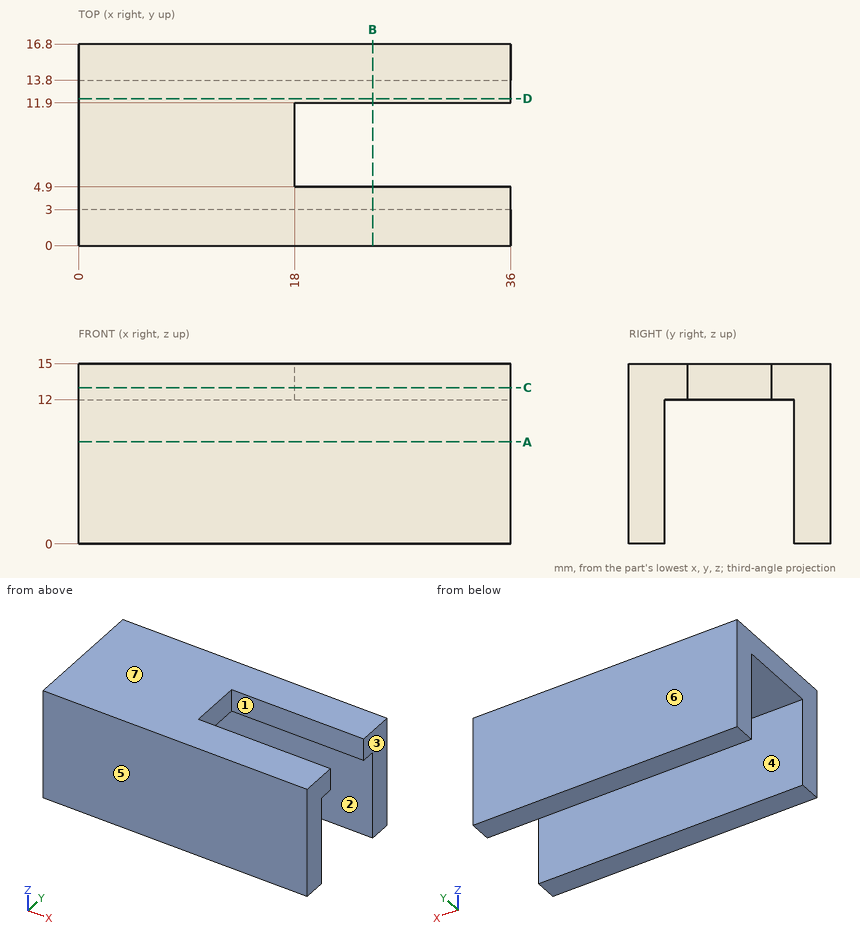
The figure shows three views and two pictorial views of one solid part (mm, origin at its lowest corner). Answer the questions. A direction names the side the tool comes from. Round coordinates to 2 decimals unless told otherwise and drop trailing zeros. Order: outer loops, then holes, each group sorted by start corner. A loop starts at its lowest first (then second) coordinate and runs counter-clockwise, first axis right, second up. Notation, with made-up numbers: (84.5, 27.25) - (93.5, 27.25) arc R11 cw to (93.5, 41.25) - close; hole circle Ø2 at (86.5, 67). An arc over 180 degrees is marked (long way). Write item = value, one per line. Start each with the question number.
1) Straight lines are drawn through the part: L1, parallel to Y at x = 33, z = 7.25; L2, parallel to Z at x = 9, y = 7.25; L3, parallel to X at y = 11.75, z = 13. For each, find the intervals that lie inside material, in ascending order.
2) Section C-C, the plane z = 13 is taken. Write down the section's boundary in (x, y).
3) Section D-D, the plane y = 12.25 is taken. Write down the section's boundary in (x, z).
4) Section B-B, the plane x = 24.5 is taken. Write down the section's boundary in (y, z).
5) Given pin 1 (1.5 mm diameter, centred on y = 7, z = 13, fed in from +X); pin 2 (1 mm diameter, centred on y = 12, z = 6, fed in from +X), each flat-ended and moving along its own axis, determine where each tip first touches the part or whether it passes through.
6) For a pull along Y with two mould halves and no side action, classify the marked faces 4, 5, 6 and 7 as released by +Y, released by -Y, zero draft, split by the parting line, or undercut.
7) For the marked faces 1, 2 and 3, determine the directions among +Z, -Z, +X, -X, +Y, -Y from which every point of the face is accessible in a straight line to the end or side of a thin tool.
8) Section A-A, the plane z = 8.5 is taken. Write down the section's boundary in (x, y), plus the area to 3 significant figures.
Results list:
q1.L1 = 0 to 3, 13.8 to 16.8
q1.L2 = 12 to 15
q1.L3 = 0 to 18
q2.outline = (0, 0) - (36, 0) - (36, 4.9) - (18, 4.9) - (18, 11.9) - (36, 11.9) - (36, 16.8) - (0, 16.8) - close
q3.outline = (0, 12) - (36, 12) - (36, 15) - (0, 15) - close
q4.outline = (0, 0) - (3, 0) - (3, 12) - (4.9, 12) - (4.9, 15) - (0, 15) - close; (11.9, 12) - (13.8, 12) - (13.8, 0) - (16.8, 0) - (16.8, 15) - (11.9, 15) - close
q5.pin_1 = 18
q5.pin_2 = through
q6.face_4 = undercut
q6.face_5 = released by -Y
q6.face_6 = released by +Y
q6.face_7 = zero draft
q7.face_1 = +Z, -Z, +X
q7.face_2 = -Z, +X, -X
q7.face_3 = +Z, -Z, +X, +Y, -Y
q8.outline = (0, 0) - (36, 0) - (36, 3) - (0, 3) - close; (0, 13.8) - (36, 13.8) - (36, 16.8) - (0, 16.8) - close
q8.area = 216 mm^2
